from build123d import *

# Parameters (mm, degrees)
SKETCH_1_W                    = 130
SKETCH_1_H                    = 30
EXTRUDE_1_DEPTH               = 6
HOLE_WIZARD_M16_1_D           = 18.8
HOLE_WIZARD_M16_1_DEPTH       = 5
HOLE_WIZARD_18_5_18_5_1_D     = 18.5
HOLE_WIZARD_18_5_18_5_1_DEPTH = 5
FILLET_1_R                    = 10


with BuildPart() as part:
    # 草图1 → 凸台-拉伸1 (new body)
    with BuildSketch(Plane(origin=(0, 0, 0), x_dir=(-1, 0, 0), z_dir=(0, 0, -1))):
        with Locations((-65, -71)):
            Rectangle(SKETCH_1_W, SKETCH_1_H)
    extrude(amount=-EXTRUDE_1_DEPTH)

    # M16 间隙孔1
    with Locations(Plane.XY.offset(6)):
        with Locations((90, -71), (115, -71)):
            Hole(HOLE_WIZARD_M16_1_D / 2, depth=HOLE_WIZARD_M16_1_DEPTH)

    # Ø18.5 (18.5) 直径孔1
    with Locations(Plane.XY.offset(6)):
        with Locations((15, -71), (40, -71), (65, -71)):
            Hole(HOLE_WIZARD_18_5_18_5_1_D / 2, depth=HOLE_WIZARD_18_5_18_5_1_DEPTH)

    # 圆角1
    fillet_1_edges = [part.edges().sort_by_distance(p)[0] for p in [
        (130, -86, 3),
        (130, -56, 3),
    ]]
    fillet(fillet_1_edges, radius=FILLET_1_R)


solid = part.part
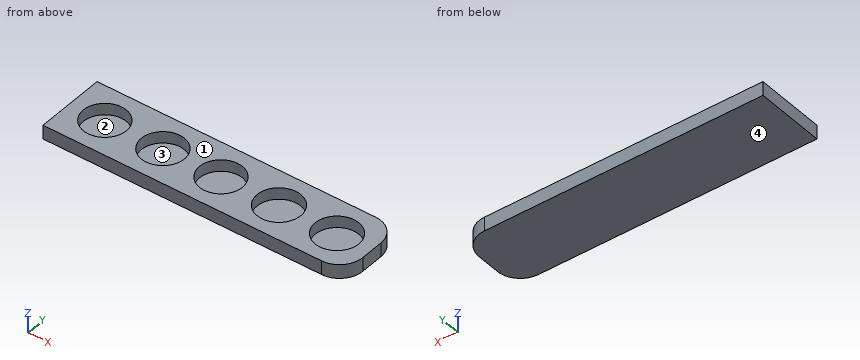
Model file for the job. Use its own axes, mm. Face numbers are marked on the shaded views. A direction names the side the tool comes from. Round coordinates to 2 decimals unless told otherwise and drop trailing zeros. Order: outer loops, then holes, each group sorted by start corner. A loop starts at its lowest first (then second) coordinate and runs counter-clockwise, first axis right, second up. Notation, with made-up numbers: M 37.25,-24 L 75.25,-24 A13 ccw 75.25,-4 Z; hole C -14,-5.75 d11. An arc over 180 degrees is marked long. Write each question's results on one line, items separated by ' | '. Start each with the question number.
(1) Probe probe 1 along Y at (x, z) = (15, 4.65); probe 2 along Y at (x, z) = (90, 4.65); probe 3 along X at (y, z) = (-75, 5.05). List the from-to ranges inside material, lowest first. Write a range as from..to.
(2) Which spindle directions (+Z, -Z, +X, -X, +Y, -Y) get a long thin tool onto all of the face, cutting with end or side? Do the marked faces 3 and 4. Say none if no direction does.
(3) Saw through at A-A, the plane z = 4.2. Give the cut face in (x, y), then the cut area to 3 significant figures.
(4) Two-plate mould, pull along X, no slides. Class the marked faces 1 and 2: pulls with the +X half, pulls with the -X half, needs draft (parallel to the pull), parting line crosses it, or undercut.
(5) Saw through at C-C, the plane y = -71. Give the cut face in (x, z).
(6) Saw through at B-B, the plane x = 65. Give the cut face in (y, z).
(7) Drop flat-ended pins along their axis: pin 1 (2 mm diameter, centred on x = 88, y = -64.5, fed in from +Z); pin 2 (1 mm diameter, centred on y = -62, z = 3, fed in from +X). Give the stop position or say it passes through.
(8) Saw through at D-D, the plane x = 90. Give the cut face in (y, z).
Established:
1) probe 1: y = -86..-80.25, -61.75..-56 | probe 2: y = -86..-80.4, -61.6..-56 | probe 3: x = 0..6.66, 23.34..31.66, 48.34..56.66, 73.34..81.49, 98.51..106.49, 123.51..130
2) face 3: +Z | face 4: -Z, +X, -X, +Y, -Y
3) outline: M 0,-86 L 120,-86 A10 ccw 130,-76 L 130,-66 A10 ccw 120,-56 L 0,-56 Z; hole C 15,-71 d18.5; hole C 40,-71 d18.5; hole C 65,-71 d18.5; hole C 90,-71 d18.8; hole C 115,-71 d18.8 | area: 2,500 mm^2
4) face 1: needs draft | face 2: undercut
5) outline: M 0,0 L 130,0 L 130,6 L 124.4,6 L 124.4,1 L 105.6,1 L 105.6,6 L 99.4,6 L 99.4,1 L 80.6,1 L 80.6,6 L 74.25,6 L 74.25,1 L 55.75,1 L 55.75,6 L 49.25,6 L 49.25,1 L 30.75,1 L 30.75,6 L 24.25,6 L 24.25,1 L 5.75,1 L 5.75,6 L 0,6 Z
6) outline: M -86,0 L -56,0 L -56,6 L -61.75,6 L -61.75,1 L -80.25,1 L -80.25,6 L -86,6 Z
7) pin 1: stops at z = 1 | pin 2: stops at x = 129.37
8) outline: M -86,0 L -56,0 L -56,6 L -61.6,6 L -61.6,1 L -80.4,1 L -80.4,6 L -86,6 Z
